Build history of the part. All positions in model axes, mm. A direction names the side the tool comes from. Round coordinates to 2 decimals unless told otherwise and drop trailing zeros. Order: outer loops, then holes, each group sorted by start corner. A loop starts at its lowest first (then second) coordinate and runs counter-clockwise, first axis right, second up. Notation, with made-up numbers: (81.5, 81) -> (132.5, 81) arc R24 ccw to (132.5, 105) -> close; hole circle Ø8 at (59, 7). An arc over 180 degrees is marked (long way). Write item = value, one per line.
from build123d import *

# Parameters (mm, degrees)
BOSS_EXTRUDE1_DEPTH = 6.35
SKETCH2_W           = 38.1
SKETCH2_H           = 41.275
SKETCH2_R           = 3.175
BOSS_EXTRUDE2_DEPTH = 3.175
SKETCH4_W           = 38.1
SKETCH4_H           = 3.175
BOSS_EXTRUDE3_DEPTH = 2.54
SKETCH5_W           = 38.1
SKETCH5_H           = 46.355
BOSS_EXTRUDE4_DEPTH = 3.175
SKETCH6_R           = 3.175
CUT_EXTRUDE1_DEPTH  = 6.35
FILLET1_R           = 5.08
SKETCH7_W           = 70.311291794
SKETCH7_H           = 15.462980338
CUT_EXTRUDE2_DEPTH  = 20.0025


with BuildPart() as part:
    # Sketch1 → Boss-Extrude1 (new body)
    with BuildSketch(Plane.XY):
        with BuildLine():
            ThreePointArc((-8.255, 0), (0, 8.255), (8.255, 0))
            Line((8.255, 0), (19.05, 0))
            ThreePointArc((19.05, 0), (0, 19.05), (-19.05, 0))
            Line((-19.05, 0), (-8.255, 0))
        make_face()
        with BuildLine():
            Line((19.05, 0), (8.255, 0))
            ThreePointArc((8.255, 0), (0, -8.255), (-8.255, 0))
            Line((-8.255, 0), (-19.05, 0))
            ThreePointArc((-19.05, 0), (0, -19.05), (19.05, 0))
        make_face()
        with BuildLine():
            Line((19.05, -45.72), (19.05, 0))
            ThreePointArc((19.05, 0), (0, -19.05), (-19.05, 0))
            Line((-19.05, 0), (-19.05, -45.72))
            Line((-19.05, -45.72), (19.05, -45.72))
        make_face()
    extrude(amount=BOSS_EXTRUDE1_DEPTH)

    # Sketch2 → Boss-Extrude2 (add)
    with BuildSketch(Plane.XZ.offset(45.72)):
        with Locations((0, 3.175)):
            Rectangle(SKETCH2_W, SKETCH2_H)
        with Locations((0, 17.4625)):
            Circle(SKETCH2_R, mode=Mode.SUBTRACT)
        with Locations((0, -11.1125)):
            Circle(SKETCH2_R, mode=Mode.SUBTRACT)
    extrude(amount=BOSS_EXTRUDE2_DEPTH)

    # Sketch4 → Boss-Extrude3 (add)
    with BuildSketch(Plane.XY.offset(23.8125)):
        with Locations((0, -47.3075)):
            Rectangle(SKETCH4_W, SKETCH4_H)
    boss_extrude3 = extrude(amount=BOSS_EXTRUDE3_DEPTH)

    # Mirror1: Boss-Extrude3 across plane
    add(boss_extrude3.mirror(Plane.XY.offset(3.175)))

    # Sketch5 → Boss-Extrude4 (add)
    with BuildSketch(Plane.XZ.offset(48.895)):
        with Locations((0, 3.175)):
            Rectangle(SKETCH5_W, SKETCH5_H)
    extrude(amount=BOSS_EXTRUDE4_DEPTH)

    # Sketch6 → Cut-Extrude1 (cut)
    with BuildSketch(Plane(origin=(0, -45.72, 0), x_dir=(1, 0, 0), z_dir=(0, 1, 0))):
        with Locations((0, 11.1125)):
            Circle(SKETCH6_R)
    cut_extrude1 = extrude(amount=-CUT_EXTRUDE1_DEPTH, mode=Mode.SUBTRACT)

    # Mirror2: Cut-Extrude1 across plane
    add(cut_extrude1.mirror(Plane.XY.offset(3.175)), mode=Mode.SUBTRACT)

    # Fillet1
    fillet1_edges = [part.edges().sort_by_distance(p)[0] for p in [
        (19.05, -48.895, 26.3525),
        (-19.05, -48.895, 26.3525),
        (-19.05, -48.895, -20.0025),
        (19.05, -48.895, -20.0025),
    ]]
    fillet(fillet1_edges, radius=FILLET1_R)

    # Sketch7 → Cut-Extrude2 (cut)
    with BuildSketch(Plane(origin=(0, 0, -20.0025), x_dir=(-1, 0, 0), z_dir=(0, 0, -1))):
        with Locations((-1.046028379, -47.628881587)):
            Rectangle(SKETCH7_W, SKETCH7_H)
    extrude(amount=-CUT_EXTRUDE2_DEPTH, mode=Mode.SUBTRACT)


solid = part.part
Q1. Probe probe 1 along Y at (x, z) = (0, 4.75) (3 decimals); probe 2 along Z at (x, y) = (0, -50.25); probe 3 along Y at (x, z) = (-7, 25.25). List the from-to ranges inside material, lowest first.
Check values:
probe_1 = -52.07 to -8.255, 8.255 to 19.05
probe_2 = 0 to 14.29, 20.64 to 26.35
probe_3 = -52.07 to -45.72
Q2. Flat gauge pins, fed straight in: pin 1 (8 mm diameter, centred on x = -15, y = 9, fed in from +Z); pin 2 (10 mm diameter, centred on y = -25.5, z = 16, fed in from +X); pin 3 (6 mm diameter, centred on x = 9.5, z = 15, fed in from +Y); pin 4 (4 mm diameter, centred on y = 8, z = 6.5, fed in from +X). Where does each tip first touch, or does it go through?
Check values:
pin_1 = 6.35
pin_2 = through
pin_3 = -45.72
pin_4 = 18.08
Q3. Cut at B-B, the plane x = 0. Give the number of separate pieces and of enclosed holes in the cut face, and give its area (3 significant figures).
Check values:
separate_pieces = 3
enclosed_holes = 0
area = 433 mm²
Q4. Which spindle directions (+Z, -Z, +X, -X, +Y, -Y) get a long thin tool onto all of the face, cutting with end or side? Do faces 4 (the face through (0, -52.07, 13)), 5 (the face through (0, -13, 6.35)). Say none if no direction does.
Check values:
face_4 = +Z, -Z, +X, -X, -Y
face_5 = +Z, +X, -X, +Y
Q5. Cut at D-D, the plane x = 4. List the corners of the cut face in (y, z), and give its area (3 significant figures).
Check values:
outline = (-52.07, 0) -> (-7.22, 0) -> (-7.22, 6.35) -> (-45.72, 6.35) -> (-45.72, 26.35) -> (-52.07, 26.35) -> close; (7.22, 0) -> (18.63, 0) -> (18.63, 6.35) -> (7.22, 6.35) -> close
area = 484 mm²
Q6. Mould opens along Y. For faces 1 (the face through (-0.41, -48.85, 20.61)), 2 (the face through (0, -45.72, 14)), 3 (the face through (-6.551, 5.023, 3.131)) say: released by +Y, released by -Y, zero draft, split by the parting line, or undercut.
Check values:
face_1 = zero draft
face_2 = released by +Y
face_3 = undercut
Q7. Cut at A-A, the plane z = 1.75. List the corners of the cut face in (x, y) (3 decimals), and give its area (3 significant figures).
Check values:
outline = (-19.05, -52.07) -> (19.05, -52.07) -> (19.05, 0) arc R19.05 ccw to (-19.05, 0) -> close; hole circle Ø16.51 at (0, 0)
area = 2,340 mm²
Q8. Cut at C-C, the plane y = 7.5. List the corners of the cut face in (x, z).
Check values:
outline = (-17.51, 0) -> (-3.45, 0) -> (-3.45, 6.35) -> (-17.51, 6.35) -> close; (3.45, 0) -> (17.51, 0) -> (17.51, 6.35) -> (3.45, 6.35) -> close
